Part model, mm, in its own coordinate system. Face numbers are marked on the shaded views. A direction names the side the tool comes from. Coordinates: 2 decimals unless noted, no trailing zeros. Write each loop counter-clockwise with the first axis right and the second up, starting at its lowest first coordinate (ties: lowest second). Pieces come first, ordered by that corner, then holes. Notation, with made-up numbers: M 22.25,-6.5 L 71.25,-6.5 A9 cw 71.25,-2.5 Z; hole C 78.25,60 d9. An arc over 180 degrees is marked long. Use a Markdown table: item, result. Add a question column.
Q1. Slice it at A-A on x = 0. Write the cut outline in (y, z).
Q2. Slice it at C-C on y = -10. Write the cut outline in (x, z), then the cut area to 3 significant figures.
Q3. Pin check, flat tips, straight feed: pin 1 Ø2 at (x, z) = (-10.5, 8) entering from +Y; pin 2 Ø1 at (x, z) = (-3, 12) entering from +Y; pin 3 Ø1.2 at (x, z) = (17, 4.5) entering from +Y; pin 4 Ø1 at (y, z) = (14, 8) entering from +X. Stop position of each tip, or through.
Q4. Tool access for the marked faces 3 and 4: list every direction of +Z, -Z, +X, -X, +Y, -Y with a clear straight run to the whole face (end or side of a thin tool).
Q5. Slice it at B-B on z = 9. Write the cut outline in (x, y), then the cut area to 3 significant figures.
Q6. Slice it at D-D on y = 1.5. Write the cut outline in (x, z), then the cut area to 3 significant figures.
Q7. Wall check: L1, parallel to Z at x = 2.5, y = -3; L2, parallel to Y at x = 0.5, z = 10; L3, parallel to X at y = -6, z = 9.25. Give the ranges that are in metal, low to high. Write a range as from..to.
Q8. Mould opens along X. For the marked faces 1 and 2 say: released by +X, released by -X, zero draft, split by the parting line, or undercut.
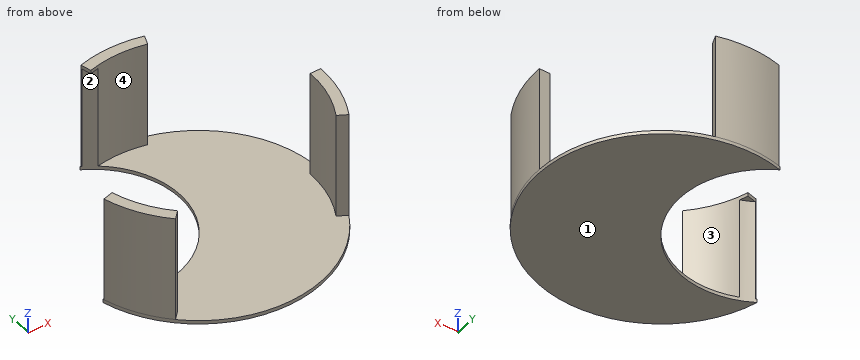
from build123d import *
from build123d.topology import SkipClean

# Parameters (mm, degrees)
SKETCH1_R           = 17.5
BOSS_EXTRUDE1_DEPTH = 0.5
BOSS_EXTRUDE2_DEPTH = 15
SKETCH3_R           = 12.279415491
CUT_EXTRUDE1_DEPTH  = 15


with BuildPart() as part:
    # Sketch1 → Boss-Extrude1 (new body)
    with BuildSketch(Plane.XY):
        Circle(SKETCH1_R)
    extrude(amount=BOSS_EXTRUDE1_DEPTH)

    # Sketch2 → Boss-Extrude2 (add)
    with SkipClean():  # the faces are left unmerged after this step: merging them gives an invalid solid
        with BuildSketch(Plane.XY.offset(0.5)):
            with BuildLine():
                ThreePointArc((15.155444566, -8.75), (16.90370196, -4.529333289), (17.5, 0))
                Line((17.5, 0), (16, 0))
                ThreePointArc((16, 0), (15.454813221, -4.141104722), (13.856406461, -8))
                Line((13.856406461, -8), (15.155444566, -8.75))
            make_face()
            with BuildLine():
                ThreePointArc((4.592982123, 16.886518742), (0.043911409, 17.499944908), (-4.508180458, 16.909355664))
                Line((-4.508180458, 16.909355664), (-4.152362122, 15.452168884))
                ThreePointArc((-4.152362122, 15.452168884), (-0.066810406, 16.000224085), (4.023175675, 15.486306593))
                Line((4.023175675, 15.486306593), (4.592982123, 16.886518742))
            make_face()
            with BuildLine():
                ThreePointArc((-15.454813221, -4.141104722), (-13.856406461, -8), (-11.313708499, -11.313708499))
                Line((-11.313708499, -11.313708499), (-12.374368671, -12.374368671))
                ThreePointArc((-12.374368671, -12.374368671), (-15.155444566, -8.75), (-16.90370196, -4.529333289))
                Line((-16.90370196, -4.529333289), (-15.454813221, -4.141104722))
            make_face()
        extrude(amount=BOSS_EXTRUDE2_DEPTH)

    # Sketch3 → Cut-Extrude1 (cut)
    with SkipClean():  # the faces are left unmerged after this step: merging them gives an invalid solid
        with BuildSketch(Plane(origin=(0, 0, 0), x_dir=(-1, 0, 0), z_dir=(0, 0, -1))):
            with Locations((10.630442789, 6.146359158)):
                Circle(SKETCH3_R)
        extrude(amount=-CUT_EXTRUDE1_DEPTH, mode=Mode.SUBTRACT)


solid = part.part
Recorded:
| question | item | result |
|---|---|---|
| 1 | outline | M -17.5,0 L 0,0 L 0,0.5 L -17.5,0.5 Z; M 12.29,0 L 17.5,0 L 17.5,15.5 L 16,15.5 L 16,0.5 L 12.29,0.5 Z |
| 2 | outline | M -14.36,0 L 14.36,0 L 14.36,0.5 L -12.49,0.5 L -12.49,15.5 L -14.36,15.5 Z |
| 2 | area | 42.4 mm² |
| 3 | pin 1 | y = -11.12 |
| 3 | pin 2 | y = 17.32 |
| 3 | pin 3 | y = 0 |
| 3 | pin 4 | through |
| 4 | face 3 | +Z, +Y |
| 4 | face 4 | +Z, -Y |
| 5 | outline | M -16.9,-4.53 A17.5 ccw -12.37,-12.37 L -11.31,-11.31 A16 cw -15.1,-5.29 A12.28 cw -16.76,-4.49 Z; M -4.51,16.91 L -4.47,16.77 A12.28 cw -2.95,15.73 A16 cw 4.02,15.49 L 4.59,16.89 A17.5 ccw Z; M 13.86,-8 L 15.16,-8.75 A17.5 ccw 17.5,0 L 16,0 A16 cw Z |
| 5 | area | 37.7 mm² |
| 6 | outline | M 0.74,0 L 17.44,0 L 17.44,0.5 L 0.74,0.5 Z |
| 6 | area | 8.35 mm² |
| 7 | L1 | 0..0.5 |
| 7 | L2 | 15.99..17.49 |
| 7 | L3 | -16.44..-14.83, 14.83..16.44 |
| 8 | face 1 | zero draft |
| 8 | face 2 | undercut |
